```python
from build123d import *

# Parameters (mm, degrees)
SKETCH1_W           = 10
SKETCH1_H           = 0.831
SKETCH1_H_2         = 1.354
SKETCH1_H_3         = 1.581
SKETCH1_H_4         = 1.737
SKETCH1_H_5         = 1.458
SKETCH1_H_6         = 0.738
SKETCH2_R           = 1.5
BOSS_EXTRUDE1_DEPTH = 17


with BuildPart() as part:
    # Sketch1 → Revolve1 (revolve)
    with BuildSketch(Plane.XY, mode=Mode.PRIVATE) as revolve1_sk:
        with Locations((5, 0.4155)):
            Rectangle(SKETCH1_W, SKETCH1_H)
        Polygon((10, 0.831), (10, 0), (20, 0), (20, 1.008), (10, 1.008), align=None)
        Polygon((20, 1.008), (20, 0), (30, 0), (30, 1.222), (20, 1.222), align=None)
        Polygon((30, 1.222), (30, 0), (40, 0), (40, 1.354), (40, 1.59), (30, 1.59), align=None)
        with Locations((45, 0.677)):
            Rectangle(SKETCH1_W, SKETCH1_H_2)
        Polygon((50, 1.354), (50, 0), (60, 0), (60, 1.783), (60, 1.867), (50, 1.867), align=None)
        Polygon((60, 1.783), (60, 0), (70, 0), (70, 1.623), (70, 1.783), align=None)
        Polygon((70, 1.623), (70, 0), (80, 0), (80, 1.581), (80, 1.623), align=None)
        with Locations((85, 0.7905)):
            Rectangle(SKETCH1_W, SKETCH1_H_3)
        Polygon((90, 1.581), (90, 0), (100, 0), (100, 1.655), (90, 1.655), align=None)
        Polygon((100, 1.655), (100, 0), (110, 0), (110, 1.737), (110, 2.092), (100, 2.092), align=None)
        with Locations((115, 0.8685)):
            Rectangle(SKETCH1_W, SKETCH1_H_4)
        Polygon((120, 1.737), (120, 0), (130, 0), (130, 1.808), (120, 1.808), align=None)
        Polygon((130, 1.808), (130, 0), (140, 0), (140, 1.826), (140, 1.957), (130, 1.957), align=None)
        Polygon((140, 1.826), (140, 0), (150, 0), (150, 1.458), (150, 1.826), align=None)
        with Locations((155, 0.729)):
            Rectangle(SKETCH1_W, SKETCH1_H_5)
        Polygon((160, 1.458), (160, 0), (170, 0), (170, 1.573), (160, 1.573), align=None)
        Polygon((170, 1.573), (170, 0), (180, 0), (180, 0.738), (180, 1.608), (170, 1.608), align=None)
        with Locations((185, 0.369)):
            Rectangle(SKETCH1_W, SKETCH1_H_6)
        Polygon((190, 0.738), (190, 0), (200, 0), (200, 2.782), (190, 2.782), align=None)
    revolve(revolve1_sk.sketch.rotate(Axis((0, 0, 0), (1, 0, 0)), 90), axis=Axis((0, 0, 0), (1, 0, 0)))

    # Sketch2 → Boss-Extrude1 (add)
    with BuildSketch(Plane.ZY):
        Circle(SKETCH2_R)
    extrude(amount=BOSS_EXTRUDE1_DEPTH)


solid = part.part
```
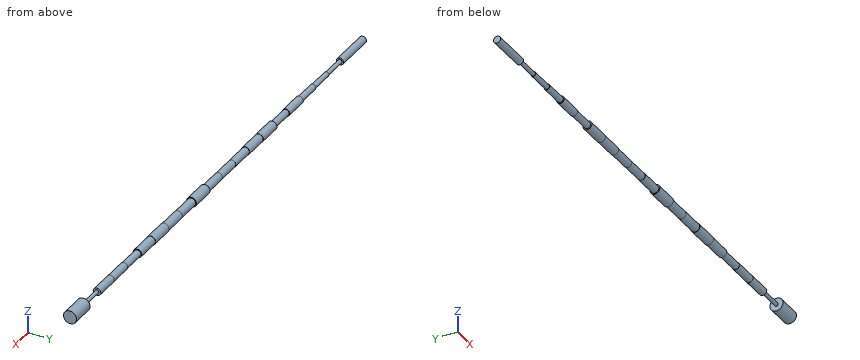
Check sheet for the modelled part. Datum: model origin and axes. Units: mm. Give positions to 0.01 mm unless a question says otherwise; leave off trailing zeros. Write each loop counter-clockwise with the first axis right and the second up, starting at its lowest first coordinate (ties: lowest second). Pieces come first, ordered by that corner, then holes.
Item 1: Cross-section at A-A (x = 57). Enter the section's corners in (y, z), and give its area (3 significant figures).
Item 2: Gauge pin test, flat ends, axial feed: pin 1 (2 mm diameter, centred on x = 123.5, y = 1, fed in from -Z); pin 2 (2 mm diameter, centred on x = 80, y = -0.5, fed in from +Z); pin 3 (1 mm diameter, centred on x = 165.5, z = 1, fed in from -Y). Record the tip position at first contact, or that the pin passes through.
Item 3: Scan lines: L1, parallel to X at y = -0.75, z = -1.05; L2, parallel to X at y = 0.1, z = -1.05; L3, parallel to Y at x = 126.5, z = -1.35. Record each from-to range of solid material in increasing order.
Report:
1. outline: circle Ø3.73 at (0, 0)
1. area: 11.0 mm2
2. pin 1: stops at z = -1.81
2. pin 2: stops at z = 1.62
2. pin 3: stops at y = -1.49
3. L1: x = -17 to 0, 30 to 180, 190 to 200
3. L2: x = -17 to 0, 20 to 180, 190 to 200
3. L3: y = -1.2 to 1.2
